```python
from build123d import *

# Parameters (mm, degrees)
F0_W      = 7
F0_H      = 31
F1_DEPTH  = 14
F2_R      = 1.35
F3_DEPTH  = 8
F4_R      = 10.2
F5_DEPTH  = 30
F6_R      = 1.35
F7_DEPTH  = 9
F8_R      = 1.5
F9_DEPTH  = 7
F10_R     = 18
F11_DEPTH = 44.001
F13_DEPTH = 31
F14_W     = 7
F14_H     = 7.299138
F14_R     = 1.35
F15_DEPTH = 2


with BuildPart() as f1:
    # F0 (on Top) → F1 (new body)
    with BuildSketch(Plane.XY):
        with Locations((-10.5, 15.5)):
            Rectangle(F0_W, F0_H)
        Polygon((-22, 31), (-14, 31), (-7, 31), (-7, 36), (7, 36), (7, 31), (14, 31), (22, 31), (22, 40), (-22, 40), align=None)
        with Locations((10.5, 15.5)):
            Rectangle(F0_W, F0_H)
    extrude(amount=F1_DEPTH)

    # F2 (on face) → F3 (cut)
    with BuildSketch(Plane.XY.offset(14)):
        with Locations((-10, 4.2)):
            Circle(F2_R)
        with Locations((-10, 30.7)):
            Circle(F2_R)
        with Locations((10, 30.7)):
            Circle(F2_R)
        with Locations((10, 4.2)):
            Circle(F2_R)
    extrude(amount=-F3_DEPTH, mode=Mode.SUBTRACT)

    # F4 (on face) → F5 (cut)
    with BuildSketch(Plane(origin=(-14, 0, 0), x_dir=(0, -1, 0), z_dir=(-1, 0, 0))):
        with Locations((-17.45, 15)):
            Circle(F4_R)
    extrude(amount=-F5_DEPTH, mode=Mode.SUBTRACT)

    # F6 (on face) → F7 (cut)
    with BuildSketch(Plane(origin=(0, 0, 0), x_dir=(1, 0, 0), z_dir=(0, 0, -1))):
        with Locations((9.5, -4.2)):
            Circle(F6_R)
        with Locations((-9.5, -4.2)):
            Circle(F6_R)
        with Locations((9.5, -26.2)):
            Circle(F6_R)
        with Locations((-9.5, -26.2)):
            Circle(F6_R)
    extrude(amount=-F7_DEPTH, mode=Mode.SUBTRACT)

    # F8 (on face) → F9 (cut)
    with BuildSketch(Plane.XZ.offset(-31)):
        with Locations((-17, 4)):
            Circle(F8_R)
        with Locations((17, 4)):
            Circle(F8_R)
    extrude(amount=-F9_DEPTH, mode=Mode.SUBTRACT)

    # F10 (on face) → F11 (cut, through all)
    with BuildSketch(Plane.YZ.offset(22)):
        with Locations((52, 18)):
            Circle(F10_R)
    extrude(amount=-F11_DEPTH, mode=Mode.SUBTRACT)

    # F12 (on face) → F13 (cut, through all)
    with BuildSketch(Plane.XZ):
        with BuildLine():
            Line((-12.9, -5.045816), (-12.9, 4))
            ThreePointArc((-12.9, 4), (-18.692576, 7.734325), (-19.70253, 0.916766))
            Line((-19.70253, 0.916766), (-12.9, -5.045816))
        make_face()
        with BuildLine():
            Line((12.9, -5.045816), (19.70253, 0.916766))
            ThreePointArc((19.70253, 0.916766), (18.692576, 7.734325), (12.9, 4))
            Line((12.9, 4), (12.9, -5.045816))
        make_face()
    extrude(amount=-F13_DEPTH, mode=Mode.SUBTRACT)

    # F14 (on face) → F15 (join)
    with BuildSketch(Plane.XY.offset(14)):
        with Locations((10.5, 3.649569)):
            Rectangle(F14_W, F14_H)
        with Locations((10, 4.2)):
            Circle(F14_R, mode=Mode.SUBTRACT)
        with Locations((-10.5, 3.649569)):
            Rectangle(F14_W, F14_H)
        with Locations((-10, 4.2)):
            Circle(F14_R, mode=Mode.SUBTRACT)
    extrude(amount=F15_DEPTH)


solid = f1.part
```
Read the model definition and answer for the solid it produces. Units are mm, in the model's axes. A direction names the side the tool comes from. Give positions to 0.01 mm unless a question says otherwise; leave off trailing zeros. Loops run counter-clockwise (first coordinate to the right, second up) from the corner with the lowest first, then second, coordinate; pieces in that order, holes last.
Item 1: The mould has two halves that part along Z. Classify faces 1 (the cylindrical face through (-12.984, 15.283, 4.827)), 2 (the flat face through (-14, 29, 10)), 3 (the flat face through (14, 32, 14)), 4 (the cylindrical face through (-18.5, 34.45, 4.07)): released by +Z, released by -Z, zero draft, split by the parting line, or undercut.
Item 2: For faces 5 (the flat face through (-15, 32, 14)), 6 (the cylindrical face through (-9.38, 29.5, 10.06)), 7 (the cylindrical face through (8.15, 4.14, 3.44)), determine the directions among +Z, -Z, +X, -X, +Y, -Y from which every point of the face is accessible in a straight line to the end or side of a thin tool.
Item 3: The part is cut by section C-C (y = 26.2). Write down the section's boundary in (x, z).
Item 4: The part is cut by section D-D (y = 4.2). Write down the section's boundary in (x, z), and give its area (3 significant figures).
Item 5: Each of these flat-tipped pins is pushed along its axis until it touches: pin 1 Ø1 at (y, z) = (25.5, 2) entering from -X; pin 2 Ø0.5 at (x, y) = (-11, 4.5) entering from +Z; pin 3 Ø3.5 at (x, y) = (10, 30.7) entering from +Z; pin 4 Ø4 at (x, y) = (15.5, 5.5) entering from +Z. Where does it stop, or does it pass through?
Item 6: The part is cut by section B-B (x = -17). Write down the section's boundary in (y, z).
Item 7: The part is cut by section A-A (z = 11). Write down the section's boundary in (x, y), and give its area (3 significant figures).
Item 8: Find the intervals of material crossed by line 1 along X through (y, z) = (26.2, 3.25); line 2 along X through (y, z) = (32.5, 6); line 3 along X through (y, z) = (28, 12.25), in increasing order.
Taken from the geometry:
1. face 1: released by -Z
1. face 2: zero draft
1. face 3: released by +Z
1. face 4: undercut
2. face 5: +Z, +X, -X, +Y
2. face 6: +Z
2. face 7: -Z
3. outline: (-14, 6.79) arc R4.1 cw to (-12.9, 4) - (-12.9, 0) - (-10.85, 0) - (-10.85, 9) - (-8.15, 9) - (-8.15, 0) - (-7, 0) - (-7, 9.76) - (-14, 9.76) - close; (7, 0) - (8.15, 0) - (8.15, 9) - (10.85, 9) - (10.85, 0) - (12.9, 0) - (12.9, 4) arc R4.1 cw to (14, 6.79) - (14, 9.76) - (7, 9.76) - close
4. outline: (-14, 6.79) arc R4.1 cw to (-12.9, 4) - (-12.9, 0) - (-10.85, 0) - (-10.85, 6) - (-11.35, 6) - (-11.35, 16) - (-14, 16) - close; (-8.65, 9) - (-8.15, 9) - (-8.15, 0) - (-7, 0) - (-7, 16) - (-8.65, 16) - close; (7, 0) - (8.15, 0) - (8.15, 9) - (8.65, 9) - (8.65, 16) - (7, 16) - close; (10.85, 0) - (12.9, 0) - (12.9, 4) arc R4.1 cw to (14, 6.79) - (14, 16) - (11.35, 16) - (11.35, 6) - (10.85, 6) - close
4. area: 122 mm2
5. pin 1: stops at x = -12.9
5. pin 2: stops at z = 6
5. pin 3: stops at z = 14
5. pin 4: stops at z = 16
6. outline: (31, 0) - (40, 0) - (40, 4.58) arc R18 cw to (34.45, 14) - (31, 14) - (31, 5.5) - (38, 5.5) - (38, 2.5) - (31, 2.5) - close
7. outline: (-22, 31) - (-14, 31) - (-14, 26.83) - (-7, 26.83) - (-7, 35.42) - (-22, 35.42) - close; (-14, 0) - (-7, 0) - (-7, 8.07) - (-14, 8.07) - close; (7, 0) - (14, 0) - (14, 8.07) - (7, 8.07) - close; (7, 26.83) - (14, 26.83) - (14, 31) - (22, 31) - (22, 35.42) - (7, 35.42) - close; hole circle Ø2.7 at (-10, 4.2); hole circle Ø2.7 at (-10, 30.7); hole circle Ø2.7 at (10, 4.2); hole circle Ø2.7 at (10, 30.7)
7. area: 281 mm2
8. line 1: x = -12.9 to -10.85, -8.15 to -7, 7 to 8.15, 10.85 to 12.9
8. line 2: x = -22 to -7, 7 to 22
8. line 3: x = -14 to -7, 7 to 14
